Verification items for this drawing (mm, ordinates from the low corner). A direction names the side the tool comes from. Round coordinates to 2 decimals unless told otherwise and drop trailing zeros. Write each loop counter-clockwise with the first axis right and the second up, starting at its lowest first coordinate (ties: lowest second). Pieces come first, ordered by that corner, then holes.
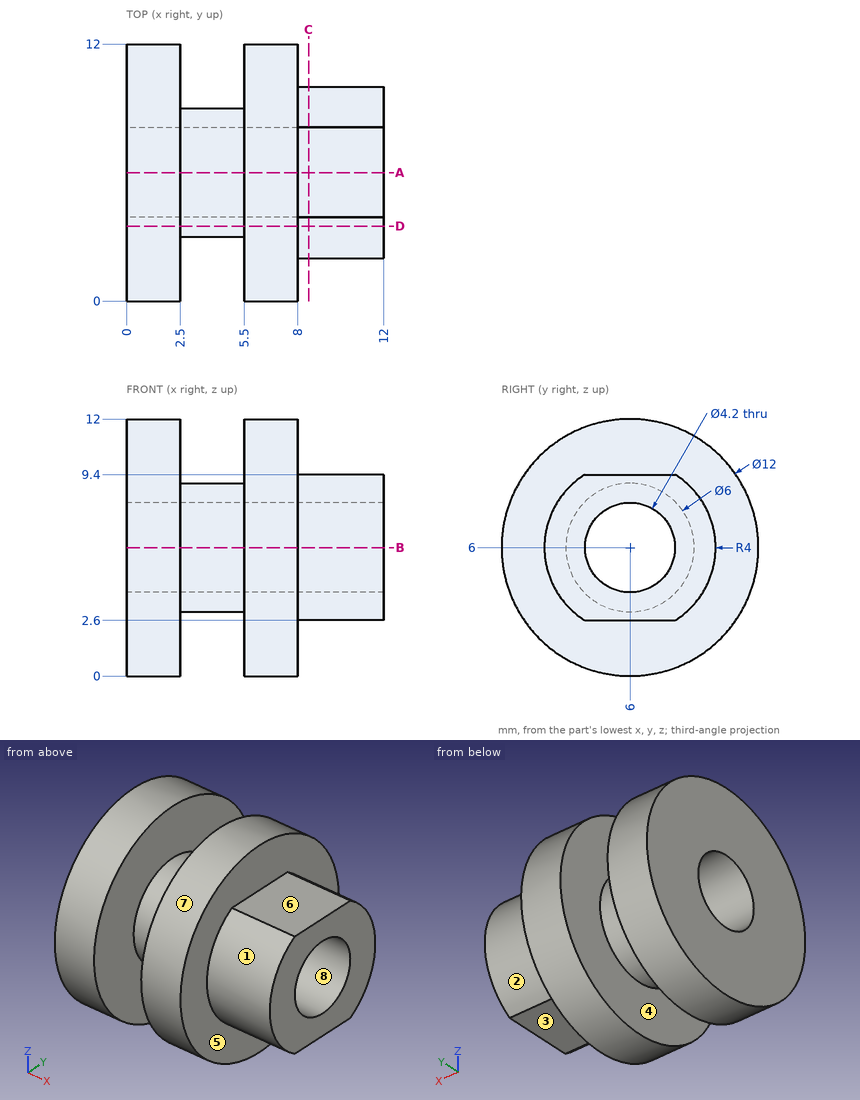
1. Depth check by flat-ended pin: pin 1 Ø4.5 at (x, y) = (9.5, 6.5) entering from -Z; pin 2 Ø3 at (x, y) = (10.5, 5) entering from +Z; pin 3 Ø1.5 at (x, z) = (5, 9) entering from -Y; pin 4 Ø1 at (y, z) = (1.5, 2.5) entering from +X. Enter the tip coordinate at first touch or a pass-through.
2. Section check D-D (y = 3.5). Record the cut outline in (x, z), plus the area to 3 significant figures.
3. Section check A-A (y = 6). Record the cut outline in (x, z), plus the area to 3 significant figures.
4. Access from +Z, -Z, +X, -X, +Y, -Y to the whole of each face (thin tool, end or side, straight path). Record for the marked faces 1, 2, 3, 4 and 5.
5. Release check for a two-part mould opening along Y. For the marked faces 6, 7 and 8 record: +Y half, -Y half, draft (parallel to the pull), parting line (faces both ways), or undercut.
6. Scan lines: line 1 along X through (y, z) = (3.5, 11.25); line 2 along Y through (x, z) = (7, 6); line 3 along X through (y, z) = (4.5, 3). Record each from-to range of solid material in increasing order.
7. Section check C-C (x = 8.5). Record the cut outline in (y, z).
8. Section check B-B (z = 6). Record the cut outline in (x, y).
Results below:
1. pin 1: stops at z = 0
1. pin 2: stops at z = 9.4
1. pin 3: stops at y = 0.52
1. pin 4: stops at x = 8
2. outline: (0, 0.55) - (2.5, 0.55) - (2.5, 4.34) - (5.5, 4.34) - (5.5, 0.55) - (8, 0.55) - (8, 2.88) - (12, 2.88) - (12, 9.12) - (8, 9.12) - (8, 11.45) - (5.5, 11.45) - (5.5, 7.66) - (2.5, 7.66) - (2.5, 11.45) - (0, 11.45) - close
2. area: 89.5 mm2
3. outline: (0, 0) - (2.5, 0) - (2.5, 3) - (5.5, 3) - (5.5, 0) - (8, 0) - (8, 2.6) - (12, 2.6) - (12, 3.9) - (0, 3.9) - close; (0, 8.1) - (12, 8.1) - (12, 9.4) - (8, 9.4) - (8, 12) - (5.5, 12) - (5.5, 9) - (2.5, 9) - (2.5, 12) - (0, 12) - close
3. area: 54.8 mm2
4. face 1: +X, -Y
4. face 2: +X, +Y
4. face 3: -Z, +X, +Y, -Y
4. face 4: none
4. face 5: +X
5. face 6: draft
5. face 7: parting line
5. face 8: undercut
6. line 1: x = 0 to 2.5, 5.5 to 8
6. line 2: y = 0 to 3.9, 8.1 to 12
6. line 3: x = 0 to 2.5, 5.5 to 12
7. outline: (3.89, 2.6) - (8.11, 2.6) arc R4 ccw to (8.11, 9.4) - (3.89, 9.4) arc R4 ccw to start; hole circle Ø4.2 at (6, 6)
8. outline: (0, 0) - (2.5, 0) - (2.5, 3) - (5.5, 3) - (5.5, 0) - (8, 0) - (8, 2) - (12, 2) - (12, 3.9) - (0, 3.9) - close; (0, 8.1) - (12, 8.1) - (12, 10) - (8, 10) - (8, 12) - (5.5, 12) - (5.5, 9) - (2.5, 9) - (2.5, 12) - (0, 12) - close
